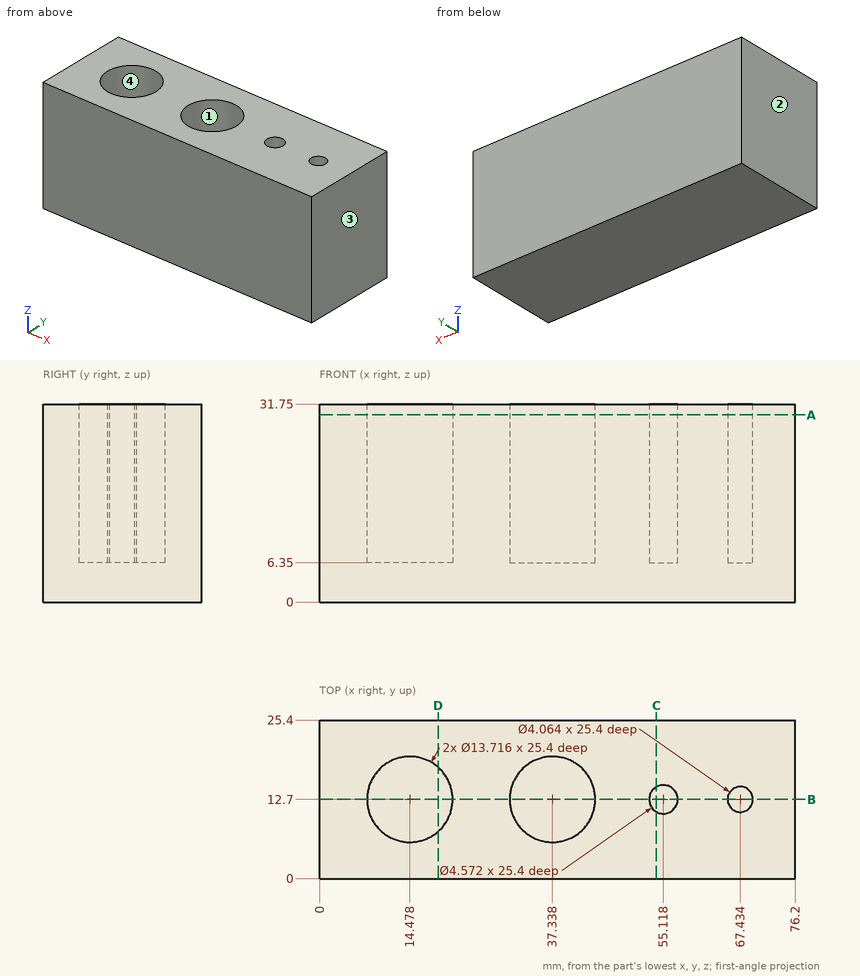
Verification items for this drawing (mm, ordinates from the low corner). Coordinates: 2 decimals unless noted, no trailing zeros. Order: outer loops, then holes, each group sorted by start corner. A loop starts at its lowest first (then second) coordinate and runs counter-clockwise, first axis right, second up. Notation, with made-up numbers: (62, -29.75) - (112, -29.75) arc R26 cw to (112, -12.75) - close; hole circle Ø2 at (48, 54). An arc over 180 degrees is marked (long way). Answer in a Markdown table with one row per item. Add a question column.
1. Gauge pin test, flat end, axial feed: pin 1 Ø1.2 at (x, y) = (68, 12) entering from +Z. Record the tip position at first contact, or that the pin passes through.
2. Section check C-C (x = 54). Enter the section's corners in (y, z).
3. Section check B-B (y = 12.7). Enter the section's corners in (x, z).
4. Section check A-A (z = 30). Enter the section's corners in (x, y), plus the area to 3 significant figures.
5. Draft check along X on the marked faces 1, 2, 3 and 4. Enter one of: +X half, -X half, draft (parallel to the pull), parting line (faces both ways), or undercut.
6. Material ranges on L1, parallel to X at y = 16, z = 17; L2, parallel to Z at x = 10.5, y = 17.25; L3, parallel to Y at x = 56, z = 28, recorded low to high. Write a range as [from, to].
7. Section check D-D (x = 19). Enter the section's corners in (y, z).
Data:
| question | item | result |
|---|---|---|
| 1 | pin 1 | stops at z = 6.35 |
| 2 | outline | (0, 0) - (25.4, 0) - (25.4, 31.75) - (14.69, 31.75) - (14.69, 6.35) - (10.71, 6.35) - (10.71, 31.75) - (0, 31.75) - close |
| 3 | outline | (0, 0) - (76.2, 0) - (76.2, 31.75) - (69.47, 31.75) - (69.47, 6.35) - (65.4, 6.35) - (65.4, 31.75) - (57.4, 31.75) - (57.4, 6.35) - (52.83, 6.35) - (52.83, 31.75) - (44.2, 31.75) - (44.2, 6.35) - (30.48, 6.35) - (30.48, 31.75) - (21.34, 31.75) - (21.34, 6.35) - (7.62, 6.35) - (7.62, 31.75) - (0, 31.75) - close |
| 4 | outline | (0, 0) - (76.2, 0) - (76.2, 25.4) - (0, 25.4) - close; hole circle Ø13.72 at (14.48, 12.7); hole circle Ø13.72 at (37.34, 12.7); hole circle Ø4.57 at (55.12, 12.7); hole circle Ø4.06 at (67.43, 12.7) |
| 4 | area | 1,610 mm² |
| 5 | face 1 | undercut |
| 5 | face 2 | -X half |
| 5 | face 3 | +X half |
| 5 | face 4 | undercut |
| 6 | L1 | x = [0, 8.47], [20.49, 31.33], [43.35, 76.2] |
| 6 | L2 | z = [0, 6.35] |
| 6 | L3 | y = [0, 10.59], [14.81, 25.4] |
| 7 | outline | (0, 0) - (25.4, 0) - (25.4, 31.75) - (17.86, 31.75) - (17.86, 6.35) - (7.54, 6.35) - (7.54, 31.75) - (0, 31.75) - close |
